Read the model definition and answer for the solid it produces. Units are mm, in the model's axes. Coordinates: 2 decimals unless noted, no trailing zeros. Loops run counter-clockwise (first coordinate to the right, second up) from the corner with the lowest first, then second, coordinate; pieces in that order, holes last. Notation, with made-up numbers: M 9,10.25 L 20,10.25 A22 ccw 20,17.25 Z; hole C 74.5,44 d11. An arc over 180 degrees is marked long. Put each result on its own line as item: value.
from build123d import *

# Parameters (mm, degrees)
SKETCH1_R           = 1.190625
BOSS_EXTRUDE1_DEPTH = 1.5875


with BuildPart() as part:
    # Sketch1 → Boss-Extrude1 (new body)
    with BuildSketch(Plane(origin=(0, 0, 0), x_dir=(1, 0, 0), z_dir=(0, 1, 0))):
        Polygon((0, 54.692295537), (0, 7.067295537), (0, 0), (39.359085702, 0), (39.359085702, 7.067295537), (39.359085702, 54.692295537), (39.359085702, 57.470420537), (0, 57.470420537), align=None)
        with Locations((2.778125, 54.692295537)):
            Circle(SKETCH1_R, mode=Mode.SUBTRACT)
        with Locations((36.580960702, 7.067295537)):
            Circle(SKETCH1_R, mode=Mode.SUBTRACT)
        with Locations((2.778125, 7.067295537)):
            Circle(SKETCH1_R, mode=Mode.SUBTRACT)
        with Locations((36.580960702, 54.692295537)):
            Circle(SKETCH1_R, mode=Mode.SUBTRACT)
        Polygon((4.7625, 52.707920537), (4.7625, 7.067295537), (4.7625, 4.7625), (34.596585702, 4.7625), (34.596585702, 7.067295537), (34.596585702, 52.707920537), align=None, mode=Mode.SUBTRACT)
    extrude(amount=BOSS_EXTRUDE1_DEPTH)


solid = part.part
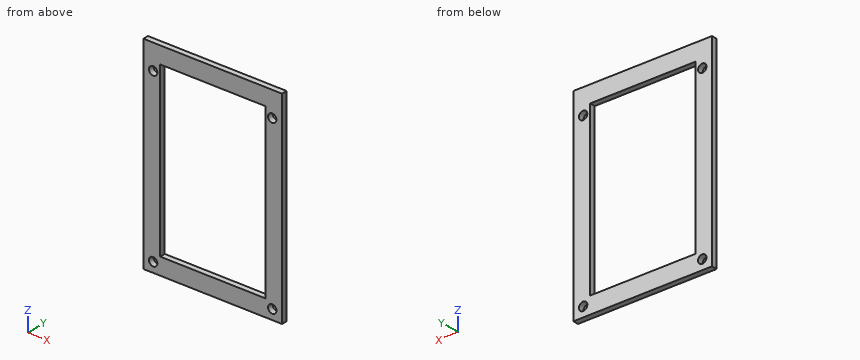
1) Find section C-C, the plane y = 0.5. Write down the section's boundary in (x, z).
Answer list:
outline: M 0,-57.47 L 39.36,-57.47 L 39.36,0 L 0,0 Z; hole C 2.78,-54.69 d2.38; hole C 2.78,-7.07 d2.38; hole M 4.76,-52.71 L 34.6,-52.71 L 34.6,-4.76 L 4.76,-4.76 Z; hole C 36.58,-54.69 d2.38; hole C 36.58,-7.07 d2.38
2) Find section B-B, the plane x = 10.5. Write down the section's boundary in (y, z).
Answer list:
outline: M 0,-57.47 L 1.59,-57.47 L 1.59,-52.71 L 0,-52.71 Z; M 0,-4.76 L 1.59,-4.76 L 1.59,0 L 0,0 Z
3) Find section A-A, the plane z = -40. Write down the section's boundary in (x, y).
Answer list:
outline: M 0,0 L 4.76,0 L 4.76,1.59 L 0,1.59 Z; M 34.6,0 L 39.36,0 L 39.36,1.59 L 34.6,1.59 Z
4) Given pin 1 Ø1.4 at (x, z) = (36.58, -7.07) entering from +Y, flat-ended and moving along its own axis, determine where the tip first touches the part or whether it passes through.
Answer list:
pin 1: passes through
5) Find section D-D, the plane x = 3. Write down the section's boundary in (y, z), plus the area to 3 significant figures.
Answer list:
outline: M 0,-57.47 L 1.59,-57.47 L 1.59,-55.86 L 0,-55.86 Z; M 0,-53.52 L 1.59,-53.52 L 1.59,-8.24 L 0,-8.24 Z; M 0,-5.9 L 1.59,-5.9 L 1.59,0 L 0,0 Z
area: 83.8 mm^2
6) Straight lines are drawn through the part: line 1 (Z direction, x = 10.5, y = 0.45); line 2 (X direction, y = 1.55, z = -34.5); line 3 (Z direction, x = 37, y = 1.55). For each, find the intervals that lie inside material, in ascending order. Write a range as [from, to].
Answer list:
line 1: z = [-57.47, -52.71], [-4.76, 0]
line 2: x = [0, 4.76], [34.6, 39.36]
line 3: z = [-57.47, -55.81], [-53.58, -8.18], [-5.95, 0]
